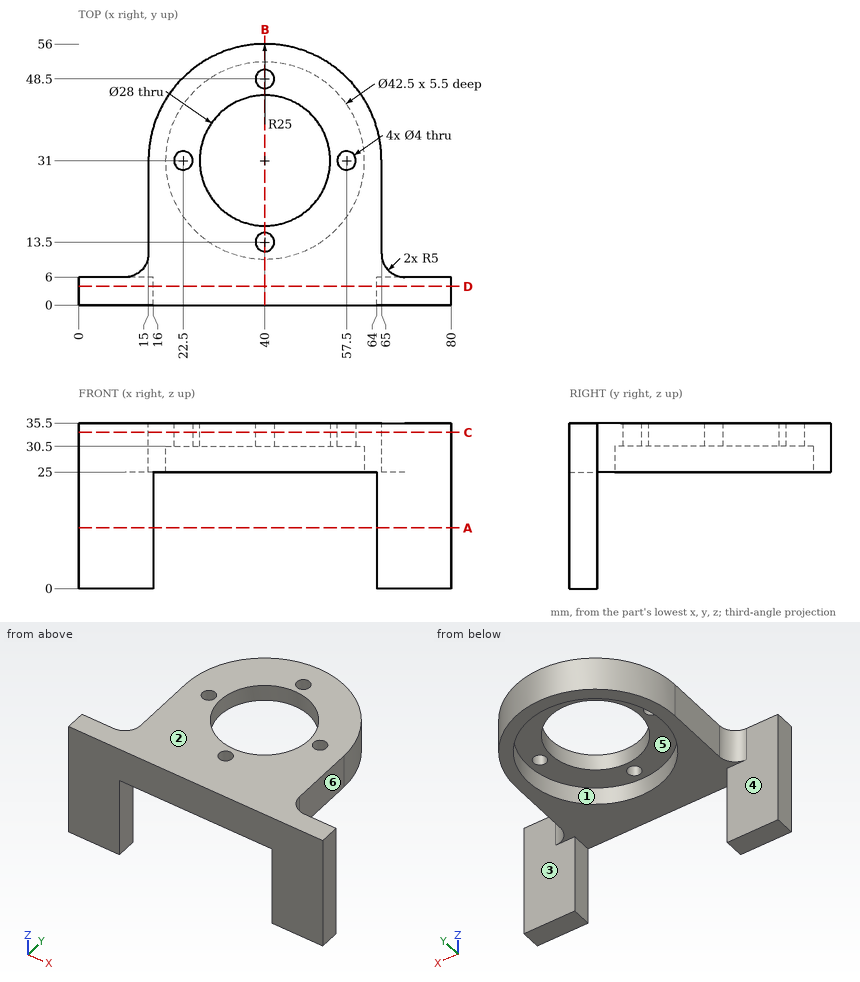
Job drawing, mm, ordinate dimensions from the low corner. One solid piece. A direction names the side the tool comes from. Coordinates: 2 decimals unless noted, no trailing zeros. Loops run counter-clockwise (first coordinate to the right, second up) from the corner with the lowest first, then second, coordinate; pieces in that order, holes last. Notation, with made-up numbers: (87.25, -6.5) - (123.25, -6.5) arc R34 cw to (123.25, 30.5) - close; hole circle Ø9 at (-36.5, 24.25). An arc over 180 degrees is marked (long way). Write item = value, one per line. Start each with the question number.
Q1. Flat gauge pins, fed straight in: pin 1 Ø3 at (x, y) = (57.5, 31) entering from +Z; pin 2 Ø17.5 at (x, z) = (71, 23) entering from +Y; pin 3 Ø11.5 at (y, z) = (23.5, 29.5) entering from +X; pin 4 Ø10 at (y, z) = (39.5, 23.5) entering from +X. Where does each tip first touch, or does it go through?
Q2. Cut at A-A, the plane z = 13. List the corners of the cut face in (x, y).
Q3. Cut at B-B, the plane x = 40. List the corners of the cut face in (y, z), then the cut area to 3 significant figures.
Q4. Cut at D-D, the plane y = 4. List the corners of the cut face in (x, z).
Q5. Cut at C-C, the plane z = 33.5. List the corners of the cut face in (x, y), then the cut area to 3 significant figures.
Q6. Drill centre lines: L1, parallel to Y at x = 40, z = 33.65; L2, parallel to Y at x = 40, z = 29.3; L3, parallel to Y at x = 74.5, z = 2. Where is each one in solid material? Low to high.
Q7. Which spindle directions (+Z, -Z, +X, -X, +Y, -Y) get a long thin tool onto all of the face, cutting with end or side? Do the marked faces 4, 5 and 6. Say none if no direction does.
Q8. Pull direction Y, two halves, no side cores. Call the marked faces 1, 2 and 3: pulls with the +Y half, pulls with the -Y half, needs draft (parallel to the pull), parting line crosses it, or undercut.
Computed:
q1.pin_1 = through
q1.pin_2 = 41.94
q1.pin_3 = 65
q1.pin_4 = 64.72
q2.outline = (0, 0) - (16, 0) - (16, 6) - (0, 6) - close; (64, 0) - (80, 0) - (80, 6) - (64, 6) - close
q3.outline = (0, 25) - (9.75, 25) - (9.75, 30.5) - (11.5, 30.5) - (11.5, 35.5) - (0, 35.5) - close; (15.5, 30.5) - (17, 30.5) - (17, 35.5) - (15.5, 35.5) - close; (45, 30.5) - (46.5, 30.5) - (46.5, 35.5) - (45, 35.5) - close; (50.5, 30.5) - (52.25, 30.5) - (52.25, 25) - (56, 25) - (56, 35.5) - (50.5, 35.5) - close
q3.area = 174 mm²
q4.outline = (0, 0) - (16, 0) - (16, 25) - (64, 25) - (64, 0) - (80, 0) - (80, 35.5) - (0, 35.5) - close
q5.outline = (0, 0) - (80, 0) - (80, 6) - (70, 6) arc R5 cw to (65, 11) - (65, 31) arc R25 ccw to (15, 31) - (15, 11) arc R5 cw to (10, 6) - (0, 6) - close; hole circle Ø4 at (22.5, 31); hole circle Ø28 at (40, 31); hole circle Ø4 at (40, 13.5); hole circle Ø4 at (40, 48.5); hole circle Ø4 at (57.5, 31)
q5.area = 2,060 mm²
q6.L1 = 0 to 11.5, 15.5 to 17, 45 to 46.5, 50.5 to 56
q6.L2 = 0 to 9.75, 52.25 to 56
q6.L3 = 0 to 6
q7.face_4 = -Z, -X, +Y
q7.face_5 = -Z
q7.face_6 = +Z, -Z, +X, +Y
q8.face_1 = undercut
q8.face_2 = needs draft
q8.face_3 = pulls with the +Y half
